Build history of the part. All positions in model axes, mm. A direction names the side the tool comes from. Round coordinates to 2 decimals unless told otherwise and drop trailing zeros. Write each loop counter-clockwise with the first axis right and the second up, starting at its lowest first coordinate (ties: lowest second). Pieces come first, ordered by that corner, then holes. Notation, with made-up numbers: (27.25, 36.5) -> (54.25, 36.5) arc R21 cw to (54.25, 75.5) -> close; hole circle Ø7 at (68.5, 21.5). An arc over 180 degrees is marked (long way). Answer as CSV lines item,"result".
from build123d import *

# Parameters (mm, degrees)
BOSS_EXTRUDE1_DEPTH = 75
CUT_EXTRUDE1_DEPTH  = 51
CUT_EXTRUDE2_DEPTH  = 36


with BuildPart() as part:
    # Sketch1 → Boss-Extrude1 (new body)
    with BuildSketch(Plane(origin=(0, 0, 0), x_dir=(0, 0, -1), z_dir=(1, 0, 0))):
        Polygon((-21.916783927, 13.855955679), (-9.869343833, 13.855955679), (28.083216073, 13.855955679), (28.083216073, -18.144044321), (-21.916783927, -18.144044321), align=None)
        Polygon((14.130656167, 37.855955679), (28.083216073, 13.855955679), (-9.869343833, 13.855955679), (-9.869343833, 37.855955679), align=None)
    extrude(amount=-BOSS_EXTRUDE1_DEPTH)

    # Sketch2 → Cut-Extrude1 (cut)
    with BuildSketch(Plane.ZY.offset(75)):
        Polygon((-28.083216073, 13.855955679), (9.869343833, 13.855955679), (9.869343833, 37.855955679), (-14.130656167, 37.855955679), align=None)
    extrude(amount=-CUT_EXTRUDE1_DEPTH, mode=Mode.SUBTRACT)

    # Sketch3 → Cut-Extrude2 (cut)
    with BuildSketch(Plane.ZY.offset(75)):
        Polygon((-19.083216073, 13.855955679), (12.916783927, 13.855955679), (-3.083216073, -2.144044321), align=None)
    extrude(amount=-CUT_EXTRUDE2_DEPTH, mode=Mode.SUBTRACT)


solid = part.part
1. Which spindle directions (+Z, -Z, +X, -X, +Y, -Y) get a long thin tool onto all of the face, cutting with end or side? Do faces 4 (the flat face through (-12, 37.856, -2)), 5 (the flat face through (-57.25, 5.97, 5.03)), 6 (the flat face through (-24, 26, -5)). Say none if no direction does.
Results found:
face 4,"+Z, -Z, +X, -X, +Y"
face 5,"-X, +Y"
face 6,"+Z, -Z, -X, +Y"
2. Drop flat-ended pins along their axis: pin 1 Ø15 at (x, z) = (-48.5, 0) entering from +Y; pin 2 Ø19 at (y, z) = (26.5, -11) entering from -X; pin 3 Ø10 at (x, y) = (-16.5, 21.5) entering from -Z. Give the stop position or say it passes through.
Results found:
pin 1,"stops at y = 8.44"
pin 2,"stops at x = -24"
pin 3,"stops at z = -26.55"
3. Cut at D-D, the plane x = -63. Write the cut outline in (y, z), then the cut area to 3 significant figures.
Results found:
outline,"(-18.14, -28.08) -> (13.86, -28.08) -> (13.86, -19.08) -> (-2.14, -3.08) -> (13.86, 12.92) -> (13.86, 21.92) -> (-18.14, 21.92) -> close"
area,"1,340 mm2"
4. Cut at C-C, the plane z = -18. Write the cut outline in (x, y), then the cut area to 3 significant figures.
Results found:
outline,"(-75, -18.14) -> (0, -18.14) -> (0, 31.2) -> (-24, 31.2) -> (-24, 13.86) -> (-39, 13.86) -> (-39, 12.77) -> (-75, 12.77) -> close"
area,"2,780 mm2"
5. Mould opens along Z. For faces 1 (the flat face through (-39, 8, -3)), 2 (the flat face through (-12, 26, 9.869)), 3 (the flat face through (-11.83, 26.02, -21.01)) say: +Z half, -Z half, draft (parallel to the pull), parting line (faces both ways), or undercut.
Results found:
face 1,"undercut"
face 2,"+Z half"
face 3,"-Z half"
6. Probe line 1 along X through (y, z) = (2, -0.5); line 2 along Y through (x, z) = (-36, -22); line 3 along X through (y, z) = (25.5, 0.5). List the from-to ranges inside material, lowest first.
Results found:
line 1,"x = -39 to 0"
line 2,"y = -18.14 to 13.86"
line 3,"x = -24 to 0"
7. Cut at B-B, the plane y = 3. Write the cut outline in (x, z).
Results found:
outline,"(-75, -28.08) -> (0, -28.08) -> (0, 21.92) -> (-75, 21.92) -> (-75, 2.06) -> (-39, 2.06) -> (-39, -8.23) -> (-75, -8.23) -> close"
8. Cut at A-A, the plane x = -5.5. Write the cut outline in (y, z).
Results found:
outline,"(-18.14, -28.08) -> (13.86, -28.08) -> (37.86, -14.13) -> (37.86, 9.87) -> (13.86, 9.87) -> (13.86, 21.92) -> (-18.14, 21.92) -> close"
